Source: three-view drawing plus pictorial views. Frame: mm from the lowest corner of the part. Round coordinates to 2 decimals unless told otherwise and drop trailing zeros. Loops run counter-clockwise (first coordinate to the right, second up) from the corner with the lowest first, then second, coordinate; pieces in that order, holes last. Notation, with made-up numbers: M -37.5,8.5 L -8.5,8.5 A27 cw -8.5,30.5 Z; hole C 61,74 d11. An arc over 180 degrees is marked long. Return JSON: item names as keys, results as strings. Group by question number.
1) Material intervals for line 1 (X direction, y = 1.3, z = 32.5); line 2 (Z direction, x = 37.5, y = 2.4); line 3 (X direction, y = 0.2, z = 32), sorted ascending. Write a range as from..to.
2) Section A-A (x = 9). Output: boundary loops of the cut face in (y, z), plus the area to 3 significant figures.
3) Section D-D (x = 37.5). Output: boundary loops of the cut face in (y, z).
4) Section C-C (y = 1.05). Output: boundary loops of the cut face in (x, z), plus the area to 3 significant figures.
5) Section B-B (z = 30). Output: boundary loops of the cut face in (x, y), plus the area to 3 significant figures.
6) Contact query for flat-ended pins moving along their axis: P1, Ø1.5, axis at x = 12, y = 0.5, coming from the -Z side (1 decimal); P2, Ø4, axis at x = 23, z = 32.5, coming from the -Y side. Output: stop coordinate, or through.
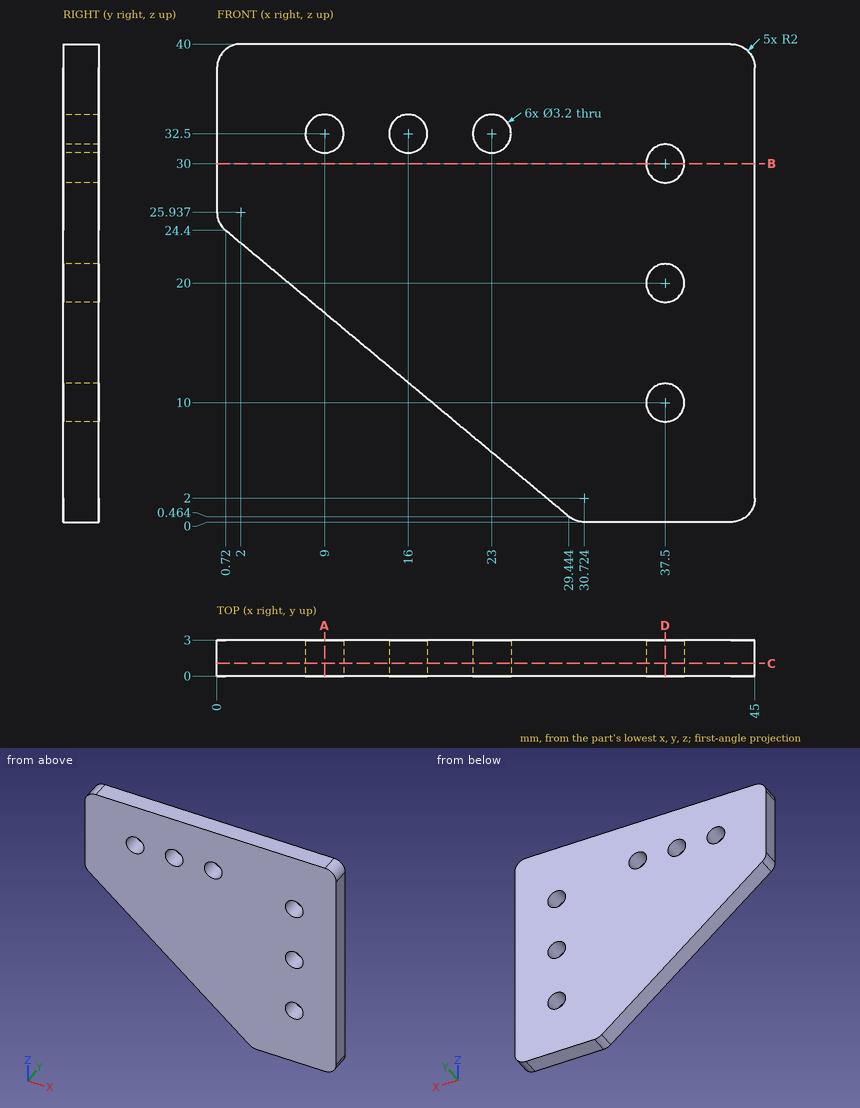
Returned:
{
 "1": {"line 1": "x = 0..7.4, 10.6..14.4, 17.6..21.4, 24.6..45", "line 2": "z = 0..8.4, 11.6..18.4, 21.6..28.4, 31.6..40", "line 3": "x = 0..7.48, 10.52..14.48, 17.52..21.48, 24.52..45"},
 "2": {"outline": "M 0,17.5 L 3,17.5 L 3,30.9 L 0,30.9 Z; M 0,34.1 L 3,34.1 L 3,40 L 0,40 Z", "area": "57.9 mm^2"},
 "3": {"outline": "M 0,0 L 3,0 L 3,8.4 L 0,8.4 Z; M 0,11.6 L 3,11.6 L 3,18.4 L 0,18.4 Z; M 0,21.6 L 3,21.6 L 3,28.4 L 0,28.4 Z; M 0,31.6 L 3,31.6 L 3,40 L 0,40 Z"},
 "4": {"outline": "M 0,25.94 A2 ccw 0.72,24.4 L 29.44,0.46 A2 ccw 30.72,0 L 43,0 A2 ccw 45,2 L 45,38 A2 ccw 43,40 L 2,40 A2 ccw 0,38 Z; hole C 9,32.5 d3.2; hole C 16,32.5 d3.2; hole C 23,32.5 d3.2; hole C 37.5,10 d3.2; hole C 37.5,20 d3.2; hole C 37.5,30 d3.2", "area": "1,370 mm^2"},
 "5": {"outline": "M 0,0 L 35.9,0 L 35.9,3 L 0,3 Z; M 39.1,0 L 45,0 L 45,3 L 39.1,3 Z", "area": "125 mm^2"},
 "6": {"P1": "stops at z = 14.4", "P2": "stops at y = 0"}
}
